Geometry: see drawing. Coordinates: mm, zero at the bounding-box minimum. A direction names the side the tool comes from. Round coordinates to 2 decimals unless told otherwise and drop trailing zeros. Loops run counter-clockwise (first coordinate to the right, second up) from the corner with the lowest first, then second, coordinate; pieces in that order, holes last. Notation, with made-up numbers: (14.25, 25) -> (67.25, 25) arc R15 ccw to (67.25, 40) -> close; hole circle Ø2 at (23.5, 59.5). An arc over 180 degrees is marked (long way). Answer in a Markdown table with one row per item.
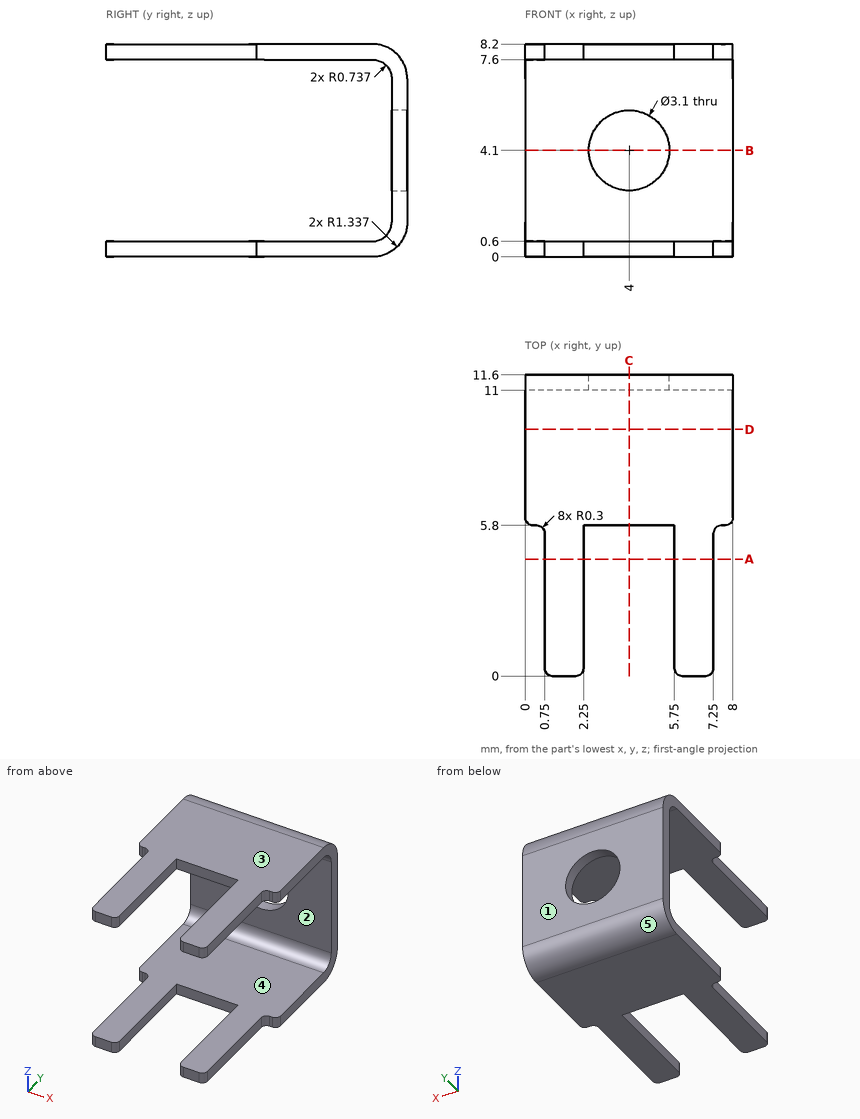
Item 1: Set-up query: the marked faces 1 and 2. Return all of +Z, -Z, +X, -X, +Y, -Y with unobstructed straight access to the full face (end or side cutting, diameter ignored); none if empty.
Ans:
| item | result |
|---|---|
| face 1 | +Z, -Z, +X, -X, +Y |
| face 2 | +X, -X, -Y |
Item 2: Section query A-A, the plane y = 4.5. Output: boundary loops of the cut face in (x, z).
Ans:
| item | result |
|---|---|
| outline | (0.75, 0) -> (2.25, 0) -> (2.25, 0.6) -> (0.75, 0.6) -> close; (0.75, 7.6) -> (2.25, 7.6) -> (2.25, 8.2) -> (0.75, 8.2) -> close; (5.75, 0) -> (7.25, 0) -> (7.25, 0.6) -> (5.75, 0.6) -> close; (5.75, 7.6) -> (7.25, 7.6) -> (7.25, 8.2) -> (5.75, 8.2) -> close |
Item 3: Section query D-D, the plane y = 9.5. Output: boundary loops of the cut face in (x, z).
Ans:
| item | result |
|---|---|
| outline | (0, 0) -> (8, 0) -> (8, 0.6) -> (0, 0.6) -> close; (0, 7.6) -> (8, 7.6) -> (8, 8.2) -> (0, 8.2) -> close |
Item 4: Mould query, pull axis Z, two halves, no side actions, for the marked faces 3, 4 and 5. Classes: released by +Z, released by -Z, zero draft, split by the parting line, or undercut.
Ans:
| item | result |
|---|---|
| face 3 | released by +Z |
| face 4 | undercut |
| face 5 | released by -Z |
Item 5: First-contact query: P1, Ø0.7, axis at y = 3, z = 8, coming from the -X side; P2, Ø0.7, axis at x = 3.5, z = 8, coming from the -Y side; P3, Ø0.7, axis at y = 3.5, z = 0.5, coming from the +X side. Flat tips, straight axial feed; report the tip coordinate or a pass-through.
Ans:
| item | result |
|---|---|
| P1 | x = 0.75 |
| P2 | y = 5.8 |
| P3 | x = 7.25 |
Item 6: Section query C-C, the plane x = 4. Output: boundary loops of the cut face in (y, z).
Ans:
| item | result |
|---|---|
| outline | (5.8, 0) -> (10.26, 0) arc R1.34 ccw to (11.6, 1.34) -> (11.6, 2.55) -> (11, 2.55) -> (11, 1.34) arc R0.74 cw to (10.26, 0.6) -> (5.8, 0.6) -> close; (5.8, 7.6) -> (10.26, 7.6) arc R0.74 cw to (11, 6.86) -> (11, 5.65) -> (11.6, 5.65) -> (11.6, 6.86) arc R1.34 ccw to (10.26, 8.2) -> (5.8, 8.2) -> close |
Item 7: Ray query, L1, parallel to X at y = 11.55, z = 4.1; L2, parallel to Z at x = 6.25, y = 6.25; L3, parallel to Y at x = 1.5, z = 5.25. Return the intervals inside material, ascending.
Ans:
| item | result |
|---|---|
| L1 | 0 to 2.45, 5.55 to 8 |
| L2 | 0 to 0.6, 7.6 to 8.2 |
| L3 | 11 to 11.6 |
Item 8: Section query B-B, the plane z = 4.1. Output: boundary loops of the cut face in (x, y).
Ans:
| item | result |
|---|---|
| outline | (0, 11) -> (2.45, 11) -> (2.45, 11.6) -> (0, 11.6) -> close; (5.55, 11) -> (8, 11) -> (8, 11.6) -> (5.55, 11.6) -> close |
